from build123d import *

# Parameters (mm, degrees)
SKETCH1_W                = 91.5
SKETCH1_H                = 122.2
BOSS_EXTRUDE1_DEPTH      = 1.5494
M3_CLEARANCE_HOLE1_D     = 3.6
M3_CLEARANCE_HOLE1_DEPTH = 12
FILLET1_R                = 3
SKETCH4_W                = 8.5
SKETCH4_H                = 88.2
SKETCH4_W_2              = 49.5
SKETCH4_H_2              = 7.5
SKETCH4_H_3              = 90.2
SKETCH4_W_3              = 67.5
SKETCH4_H_4              = 15
BOSS_EXTRUDE2_DEPTH      = 13


with BuildPart() as part:
    # Sketch1 → Boss-Extrude1 (new body)
    with BuildSketch(Plane(origin=(0, 0, 0), x_dir=(1, 0, 0), z_dir=(0, 1, 0))):
        Rectangle(SKETCH1_W, SKETCH1_H)
    extrude(amount=BOSS_EXTRUDE1_DEPTH)

    # M3 Clearance Hole1
    with Locations(Plane(origin=(0, 1.5494, 0), x_dir=(1, 0, 0), z_dir=(0, 1, 0))):
        with Locations((-40.7, 55.9), (40.7, -55.9), (40.7, 55.9), (-40.7, -55.9)):
            Hole(M3_CLEARANCE_HOLE1_D / 2, depth=M3_CLEARANCE_HOLE1_DEPTH)

    # Fillet1
    fillet1_edges = [part.edges().sort_by_distance(p)[0] for p in [
        (-45.75, 0.7747, -61.1),
        (45.75, 0.7747, -61.1),
        (45.75, 0.7747, 61.1),
        (-45.75, 0.7747, 61.1),
    ]]
    fillet(fillet1_edges, radius=FILLET1_R)

    # Sketch4 → Boss-Extrude2 (add)
    with BuildSketch(Plane.XZ):
        with Locations((41.3, -6)):
            Rectangle(SKETCH4_W, SKETCH4_H)
        with Locations((-6, -57.15)):
            Rectangle(SKETCH4_W_2, SKETCH4_H_2)
        with Locations((-41.3, -5)):
            Rectangle(SKETCH4_W, SKETCH4_H_3)
        with Locations((0, 53.4)):
            Rectangle(SKETCH4_W_3, SKETCH4_H_4)
    extrude(amount=BOSS_EXTRUDE2_DEPTH)


solid = part.part
Read the model definition and answer for the solid it produces. Units are mm, in the model's axes. A direction names the side the tool comes from. Round coordinates to 2 decimals unless told otherwise and drop trailing zeros. Write each loop counter-clockwise with the first axis right and the second up, starting at its lowest first coordinate (ties: lowest second). Pieces come first, ordered by that corner, then holes. Notation, with made-up numbers: M -15.5,1 L 10.5,1 A7 cw 10.5,14 Z; hole C -20.75,60 d5. An arc over 180 degrees is marked long. Use a Markdown table: item, result.
1) For a pull along Z with two mould halves and no side action, classify faces 1 (the flat face through (-6, -6, -60.9)), 2 (the cylindrical face through (39.732, 0.764, 54.382)), 3 (the flat face through (-1, 1.549, -1)) as pulls with the +Z half, pulls with the -Z half, needs draft (parallel to the pull), parting line crosses it, or undercut.
Answers follow:
| item | result |
|---|---|
| face 1 | pulls with the -Z half |
| face 2 | undercut |
| face 3 | needs draft |
2) Straight lines are drawn through the part: line 1 along Z through (x, y) = (40.7, 0.65); line 2 along X through (y, z) = (0.45, -55.9); line 3 along X through (y, z) = (-2.75, 16). For each, find the intervals that lie inside material, in ascending order. Write a range as [from, to].
Answers follow:
| item | result |
|---|---|
| line 1 | z = [-61.1, -57.7], [-54.1, 54.1], [57.7, 61.1] |
| line 2 | x = [-45.75, -42.5], [-38.9, 38.9], [42.5, 45.75] |
| line 3 | x = [-45.55, -37.05], [37.05, 45.55] |
3) The part is cut by section B-B (x = 40.7). Write down the section's boundary in (y, z), plus the area to 3 significant figures.
Answers follow:
| item | result |
|---|---|
| outline | M -13,-50.1 L 0,-50.1 L 0,-54.1 L 1.55,-54.1 L 1.55,54.1 L 0,54.1 L 0,38.1 L -13,38.1 Z; M 0,-61.1 L 1.55,-61.1 L 1.55,-57.7 L 0,-57.7 Z; M 0,57.7 L 1.55,57.7 L 1.55,61.1 L 0,61.1 Z |
| area | 1,320 mm2 |
4) A tool of negligible diameter and unlimited length cuts with its end or side. For faces 4 (the flat face through (-37.05, -6, -6)), 5 (the flat face through (0, -6, 45.9)), 6 (the flat face through (0, -6, 60.9)), 7 (the flat face through (41, -6, -50.1)), 8 (the flat face through (33.75, -6, 53)), from which of +Z, -Z, +X, -X, +Y, -Y can it reach the whole face along a straight path? Write none if from no direction.
Answers follow:
| item | result |
|---|---|
| face 4 | +Z, -Z, -Y |
| face 5 | +X, -X, -Y |
| face 6 | +Z, +X, -X, -Y |
| face 7 | -Z, +X, -X, -Y |
| face 8 | +Z, -Z, +X, -Y |
5) The part is cut by section D-D (z = -26.5). Write down the section's boundary in (x, y), plus the area to 3 significant figures.
Answers follow:
| item | result |
|---|---|
| outline | M -45.75,0 L -45.55,0 L -45.55,-13 L -37.05,-13 L -37.05,0 L 37.05,0 L 37.05,-13 L 45.55,-13 L 45.55,0 L 45.75,0 L 45.75,1.55 L -45.75,1.55 Z |
| area | 363 mm2 |
6) The part is cut by section A-A (z = 55.9). Write down the section's boundary in (x, y), plus the area to 3 significant figures.
Answers follow:
| item | result |
|---|---|
| outline | M -45.75,0 L -42.5,0 L -42.5,1.55 L -45.75,1.55 Z; M -38.9,0 L -33.75,0 L -33.75,-13 L 33.75,-13 L 33.75,0 L 38.9,0 L 38.9,1.55 L -38.9,1.55 Z; M 42.5,0 L 45.75,0 L 45.75,1.55 L 42.5,1.55 Z |
| area | 1,010 mm2 |
7) The part is cut by section C-C (y = -6.75). Write down the section's boundary in (x, z).
Answers follow:
| item | result |
|---|---|
| outline | M -45.55,-50.1 L -37.05,-50.1 L -37.05,40.1 L -45.55,40.1 Z; M -33.75,45.9 L 33.75,45.9 L 33.75,60.9 L -33.75,60.9 Z; M -30.75,-60.9 L 18.75,-60.9 L 18.75,-53.4 L -30.75,-53.4 Z; M 37.05,-50.1 L 45.55,-50.1 L 45.55,38.1 L 37.05,38.1 Z |
8) Flat-ended cylindrical pins translate along their axes: pin 1 (1.5 mm diameter, centred on x = -36.5, y = -11.5, fed in from -Z); pin 2 (8 mm diameter, centred on x = -15, z = 21, fed in from -Y); pin 3 (7 mm diameter, centred on x = -41.5, y = -5.5, fed in from +Z). Find the tip coordinate at first contact, or state that the pin passes through.
Answers follow:
| item | result |
|---|---|
| pin 1 | stops at z = -50.1 |
| pin 2 | stops at y = 0 |
| pin 3 | stops at z = 40.1 |
